Here's how the part is built. I have some questions about the finished solid (model axes, mm). Round coordinates to 2 decimals unless told otherwise and drop trailing zeros. Write each loop counter-clockwise with the first axis right and the second up, starting at its lowest first coordinate (ties: lowest second). Pieces come first, ordered by that corner, then holes. Notation, with made-up numbers: (-31.75, 71) - (9.25, 71) arc R14 cw to (9.25, 97) - close; hole circle Ø9 at (39, 68). An arc over 180 degrees is marked (long way). One line per item, written item: value. Start each with the question number.
Item 1: Imagine slicing it at A-A, the plane y = -2.54. Please give me the cut outline in (x, z) (3 decimals), then the cut area to 3 significant figures.
Item 2: If I drill on line 1 (Z direction, x = 4.5, y = 22.86); line 2 (Z direction, x = 8.75, y = -4), over which ranges is the centre line in solid material (lowest first)?
Item 3: Imagine slicing it at B-B, the plane z = 25.4. Please give me the cut outline in (x, y) (3 decimals).
```python
from build123d import *

# Parameters (mm, degrees)
SKETCH1_W           = 19.05
SKETCH1_H           = 127
BOSS_EXTRUDE1_DEPTH = 254
SKETCH2_R           = 2.38125
CUT_EXTRUDE1_DEPTH  = 263.509337929


with BuildPart() as part:
    # Sketch1 → Boss-Extrude1 (new body)
    with BuildSketch(Plane.XY):
        Rectangle(SKETCH1_W, SKETCH1_H)
    extrude(amount=BOSS_EXTRUDE1_DEPTH)

    # Sketch2 → Cut-Extrude1 (cut, through all)
    with BuildSketch(Plane.ZY.offset(9.525)):
        with Locations(Location((25.4, 22.86, 0), (0, 0, 270))):
            Circle(SKETCH2_R)
        with Locations(Location((25.4, -2.54, 0), (0, 0, 270))):
            Circle(SKETCH2_R)
    extrude(amount=-CUT_EXTRUDE1_DEPTH, mode=Mode.SUBTRACT)


solid = part.part
```
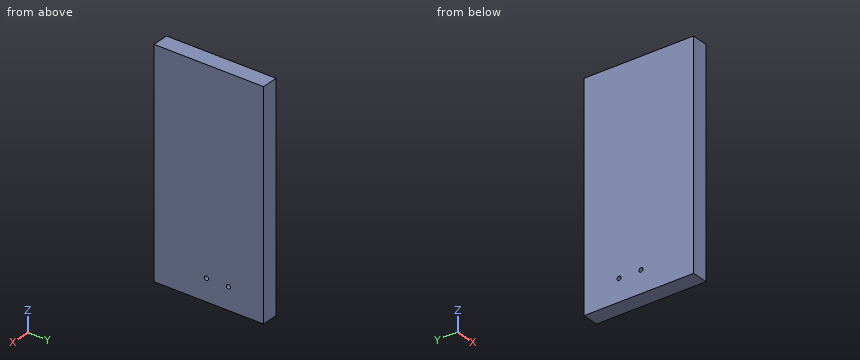
Values follow:
1. outline: (-9.525, 0) - (9.525, 0) - (9.525, 23.019) - (-9.525, 23.019) - close; (-9.525, 27.781) - (9.525, 27.781) - (9.525, 254) - (-9.525, 254) - close
1. area: 4,750 mm^2
2. line 1: z = 0 to 23.02, 27.78 to 254
2. line 2: z = 0 to 23.52, 27.28 to 254
3. outline: (-9.525, -63.5) - (9.525, -63.5) - (9.525, -4.921) - (-9.525, -4.921) - close; (-9.525, -0.159) - (9.525, -0.159) - (9.525, 20.479) - (-9.525, 20.479) - close; (-9.525, 25.241) - (9.525, 25.241) - (9.525, 63.5) - (-9.525, 63.5) - close
